from build123d import *

# Parameters (mm, degrees)
F0_W     = 50
F0_H     = 100
F0_W_2   = 40.000004
F0_H_2   = 90.000004
F1_DEPTH = 890
F2_R     = 3
F3_R     = 6


with BuildPart() as f1:
    # F0 (on Right) → F1 (new body, symmetric)
    with BuildSketch(Plane.YZ):
        Rectangle(F0_W, F0_H)
        Rectangle(F0_W_2, F0_H_2, mode=Mode.SUBTRACT)
    extrude(amount=F1_DEPTH, both=True)

    # F2
    f2_edges = [f1.edges().sort_by_distance(p)[0] for p in [
        (0, 20.000002, 45.000002),
        (0, 20.000002, -45.000002),
        (0, -20.000002, -45.000002),
        (0, -20.000002, 45.000002),
    ]]
    fillet(f2_edges, radius=F2_R)

    # F3
    f3_edges = [f1.edges().sort_by_distance(p)[0] for p in [
        (0, 25, -50),
        (0, 25, 50),
        (0, -25, 50),
        (0, -25, -50),
    ]]
    fillet(f3_edges, radius=F3_R)


solid = f1.part
For this review, take the finished solid that the model builds, in its own axes (mm). A direction names the side the tool comes from. Round coordinates to 2 decimals unless told otherwise and drop trailing zeros. Loops run counter-clockwise (first coordinate to the right, second up) from the corner with the lowest first, then second, coordinate; pieces in that order, holes last. Notation, with made-up numbers: (26, 16) - (57, 16) arc R3 ccw to (57, 20) - close; hole circle Ø1 at (35.25, 56.5). An arc over 180 degrees is marked (long way). Use one line per item in the form item = value.
1) We need section B-B on y = 7. Write out the cut boundary in (x, z).
Solutions:
outline = (-890, -50) - (890, -50) - (890, -45) - (-890, -45) - close; (-890, 45) - (890, 45) - (890, 50) - (-890, 50) - close
2) We need section C-C on x = -540. Write out the cut boundary in (y, z), then the cut area to 3 significant figures.
Solutions:
outline = (-25, -44) arc R6 ccw to (-19, -50) - (19, -50) arc R6 ccw to (25, -44) - (25, 44) arc R6 ccw to (19, 50) - (-19, 50) arc R6 ccw to (-25, 44) - close; hole (-20, -42) arc R3 ccw to (-17, -45) - (17, -45) arc R3 ccw to (20, -42) - (20, 42) arc R3 ccw to (17, 45) - (-17, 45) arc R3 ccw to (-20, 42) - close
area = 1,380 mm2
3) Wall thickness on probe 1 along Z at (x, y) = (-241, -11.5); probe 2 along Y at (x, z) = (473, -30.5): over which ranges is each line inside the solid? List them lowest first.
Solutions:
probe_1 = -50 to -45, 45 to 50
probe_2 = -25 to -20, 20 to 25
4) Clearance check with a flat-ended pin moving along its axis: P1, Ø5, axis at y = -19.5, z = 1.5, coming from the +X side. State where the tip first meets the part, or that it passes through.
Solutions:
P1 = 890
5) We need section A-A on z = -20.5. Write out the cut boundary in (x, y).
Solutions:
outline = (-890, -25) - (890, -25) - (890, -20) - (-890, -20) - close; (-890, 20) - (890, 20) - (890, 25) - (-890, 25) - close
6) Tool access review of faces 1 (the face through (12, -25, -1)), 2 (the face through (12, 0, -45)): name each direction out of +Z, -Z, +X, -X, +Y, -Y from which nothing blocks a thin tool from reaching the whole face with its end or side.
Solutions:
face_1 = +Z, -Z, +X, -X, -Y
face_2 = +X, -X
7) Mouldability with a two-part tool opening along Y and no side actions: class faces 3 (the face through (12, -20, -1)), 4 (the face through (12, 0, 50)), 5 (the face through (12, 25, -1)), 6 (the face through (12, 0, 45)) as pulls with the +Y half, pulls with the -Y half, needs draft (parallel to the pull), parting line crosses it, or undercut.
Solutions:
face_3 = undercut
face_4 = needs draft
face_5 = pulls with the +Y half
face_6 = undercut
